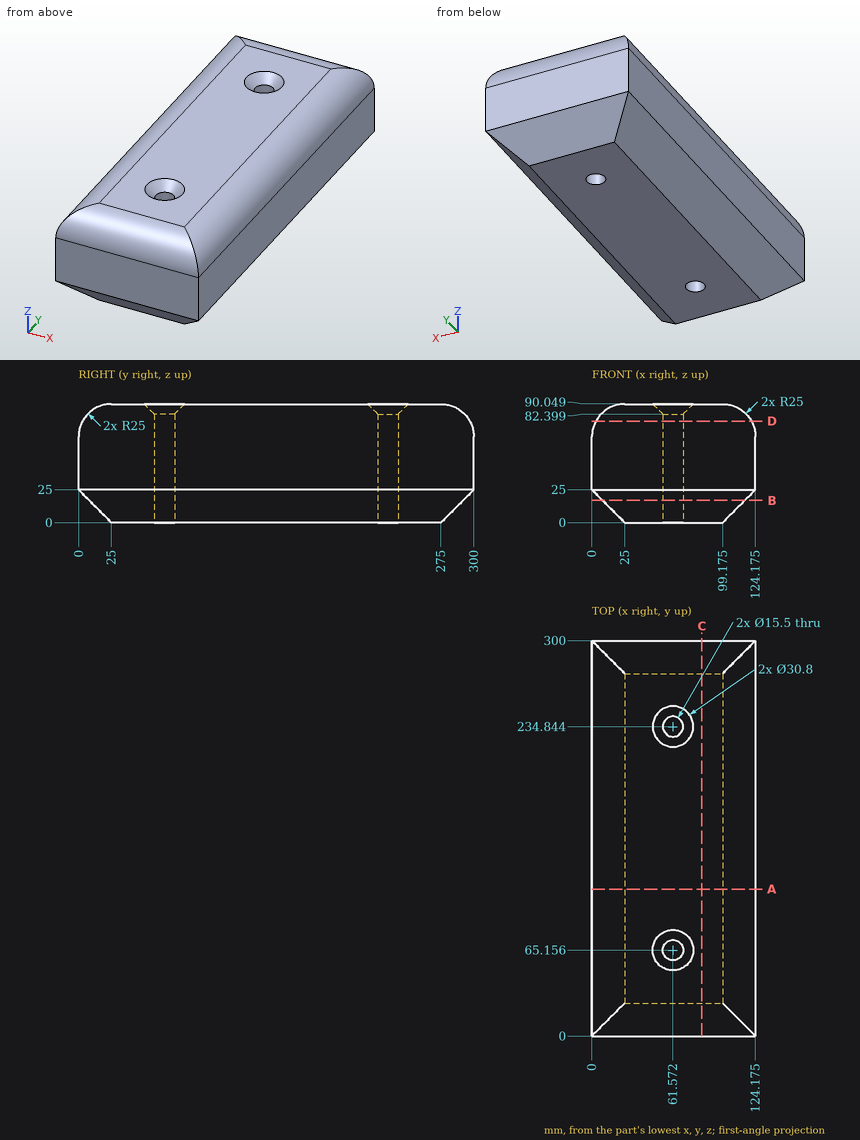
Here's the drawing with two shaded views (mm, measured from the low corner). I have some questions. Round coordinates to 2 decimals unless told otherwise and drop trailing zeros. Loops run counter-clockwise (first coordinate to the right, second up) from the corner with the lowest first, then second, coordinate; pieces in that order, holes last. Notation, with made-up numbers: M 82.5,19 L 140.5,19 A17 ccw 140.5,50 Z; hole C 24,29.5 d4. An arc over 180 degrees is marked long. Answer as CSV lines item,"result".
1) Imagine slicing it at D-D on z = 77. List the corners of the cut face in (x, y) for me.
From the geometry:
outline,"M 3.04,3.04 L 121.13,3.04 L 121.13,296.96 L 3.04,296.96 Z; hole C 61.57,65.16 d15.5; hole C 61.57,234.84 d15.5"
2) Imagine slicing it at C-C on x = 83.5. List the corners of the cut face in (y, z) for me, and give its area (3 significant figures).
From the geometry:
outline,"M 0,25 L 25,0 L 275,0 L 300,25 L 300,65.05 A25 ccw 275,90.05 L 25,90.05 A25 ccw 0,65.05 Z"
area,"26,100 mm^2"
3) Imagine slicing it at B-B on z = 17. Count the separate pieces of the cut face and the enclosed holes in it, and give its area (3 significant figures).
From the geometry:
separate pieces,"1"
enclosed holes,"2"
area,"30,300 mm^2"
4) For pin 1 Ø5 at (x, z) = (31.5, 78) entering from +Y; pin 2 Ø6 at (y, z) = (185, 15) entering from +X (1 decimal); pin 3 Ø14 at (x, y) = (61.57, 234.84) entering from +Z; pin 4 Ø1.5 at (x, z) = (86.5, 79) entering from -Y, each with a flat end and sliding along its axis, tell me the tip position at first contact or that it passes through.
From the geometry:
pin 1,"y = 297.71"
pin 2,"x = 117.2"
pin 3,"through"
pin 4,"y = 3.77"
5) If I drill on probe 1 along Y at (x, z) = (65.5, 73.5) (1 decimal); probe 2 along Y at (x, z) = (61.5, 74.5) (1 decimal); probe 3 along X at (y, z) = (13, 23) (1 decimal), over which ranges is the centre line in solid material (lowest first)?
From the geometry:
probe 1,"1.5 to 58.5, 71.8 to 228.2, 241.5 to 298.5"
probe 2,"1.9 to 57.4, 72.9 to 227.1, 242.6 to 298.1"
probe 3,"2 to 122.2"
6) Imagine slicing it at A-A on y = 111.5. List the corners of the cut face in (x, z) for me (1 decimal).
From the geometry:
outline,"M 0,25 L 25,0 L 99.2,0 L 124.2,25 L 124.2,65 A25 ccw 99.2,90 L 25,90 A25 ccw 0,65 Z"
